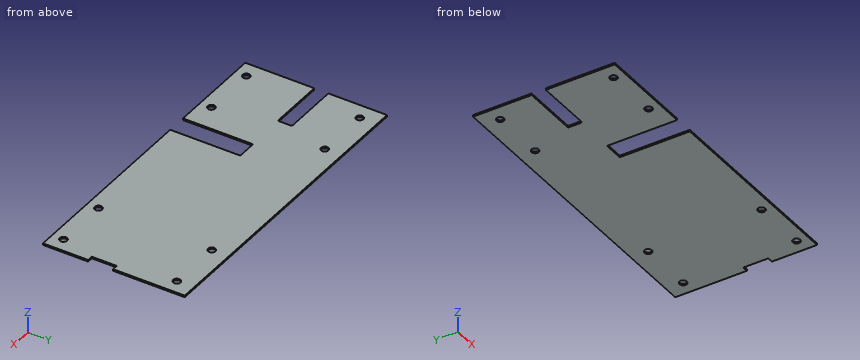
```python
from build123d import *

# Parameters (mm, degrees)
ESQUISSE1_W             = 555
ESQUISSE1_H             = 250
ESQUISSE1_R             = 6.5
BOSS_EXTRU_1_DEPTH      = 3
ESQUISSE4_W             = 100
ESQUISSE4_H             = 25
ESQUISSE4_W_2           = 35
ESQUISSE4_H_2           = 123.628962184
ESQUISSE4_W_3           = 10
ESQUISSE4_H_3           = 44
ENL_V_MAT_EXTRU_3_DEPTH = 10
CONG_1_R                = 2


with BuildPart() as part:
    # Esquisse1 → Boss.-Extru.1 (new body)
    with BuildSketch(Plane.XY):
        Rectangle(ESQUISSE1_W, ESQUISSE1_H)
        with Locations((156.5, 95)):
            Circle(ESQUISSE1_R, mode=Mode.SUBTRACT)
        with Locations((252.5, 95)):
            Circle(ESQUISSE1_R, mode=Mode.SUBTRACT)
        with Locations((156.5, -105)):
            Circle(ESQUISSE1_R, mode=Mode.SUBTRACT)
        with Locations((252.5, -105)):
            Circle(ESQUISSE1_R, mode=Mode.SUBTRACT)
        with Locations((-153.5, -105)):
            Circle(ESQUISSE1_R, mode=Mode.SUBTRACT)
        with Locations((-153.5, 95)):
            Circle(ESQUISSE1_R, mode=Mode.SUBTRACT)
        with Locations((-249.5, 95)):
            Circle(ESQUISSE1_R, mode=Mode.SUBTRACT)
        with Locations((-249.5, -105)):
            Circle(ESQUISSE1_R, mode=Mode.SUBTRACT)
    extrude(amount=BOSS_EXTRU_1_DEPTH)

    # Esquisse4 → Enlèv. mat.-Extru.3 (cut)
    with BuildSketch(Plane.XY.offset(3)):
        with Locations((-227.5, 9.128962184)):
            Rectangle(ESQUISSE4_W, ESQUISSE4_H)
        with Locations((-89, -63.185518908)):
            Rectangle(ESQUISSE4_W_2, ESQUISSE4_H_2)
        with Locations((272.5, -23.371037816)):
            Rectangle(ESQUISSE4_W_3, ESQUISSE4_H_3)
    extrude(amount=-ENL_V_MAT_EXTRU_3_DEPTH, mode=Mode.SUBTRACT)

    # Congé1
    cong_1_edges = [part.edges().sort_by_distance(p)[0] for p in [
        (-177.5, 21.628962184, 1.5),
        (-177.5, -3.371037816, 1.5),
        (-106.5, -1.371037816, 1.5),
        (-71.5, -1.371037816, 1.5),
    ]]
    fillet(cong_1_edges, radius=CONG_1_R)


solid = part.part
```
Geometry: final body of the model. Coordinates: model frame, mm. Give positions to 0.01 mm unless a question says otherwise; leave off trailing zeros. Loops run counter-clockwise (first coordinate to the right, second up) from the corner with the lowest first, then second, coordinate; pieces in that order, holes last. Notation, with made-up numbers: (84.25, 83.5) - (136.25, 83.5) arc R13 cw to (136.25, 93.5) - close; hole circle Ø3 at (20, -32). An arc over 180 degrees is marked (long way). Answer as CSV lines item,"result". Start each with the question number.
(1) Pin query (flat end, axial travel): P1, Ø0.9, axis at y = -23.5, z = 1, coming from the +X side. Return the tip coordinate at first contact, or that it passes through.
(2) Section query A-A (x = 252.5). Output: boundary loops of the cut face in (y, z).
(3) Ray query, line 1 along Y through (x, z) = (-153.5, 1.3); line 2 along Y through (x, z) = (-213.5, 0.9); line 3 along X through (y, z) = (-88, 2.6). Return the intervals inside material, ascending. Write a range as [from, to].
(4) Section query D-D (z = 0.75). Give the number of separate pieces and of enclosed holes in the cut face, and give its area (3 significant figures).
(5) Section query C-C (x = -211.5). Output: boundary loops of the cut face in (y, z), and give its area (3 significant figures).
(6) Section query B-B (y = 95). Output: boundary loops of the cut face in (x, z), and give its area (3 significant figures).
Worked answers:
1,P1,"stops at x = 267.5"
2,outline,"(-125, 0) - (-111.5, 0) - (-111.5, 3) - (-125, 3) - close; (-98.5, 0) - (88.5, 0) - (88.5, 3) - (-98.5, 3) - close; (101.5, 0) - (125, 0) - (125, 3) - (101.5, 3) - close"
3,line 1,"y = [-125, -111.5], [-98.5, 88.5], [101.5, 125]"
3,line 2,"y = [-125, -3.37], [21.63, 125]"
3,line 3,"x = [-277.5, -106.5], [-71.5, 277.5]"
4,separate pieces,"1"
4,enclosed holes,"8"
4,area,"130,000 mm^2"
5,outline,"(-125, 0) - (-3.37, 0) - (-3.37, 3) - (-125, 3) - close; (21.63, 0) - (125, 0) - (125, 3) - (21.63, 3) - close"
5,area,"675 mm^2"
6,outline,"(-277.5, 0) - (-256, 0) - (-256, 3) - (-277.5, 3) - close; (-243, 0) - (-160, 0) - (-160, 3) - (-243, 3) - close; (-147, 0) - (150, 0) - (150, 3) - (-147, 3) - close; (163, 0) - (246, 0) - (246, 3) - (163, 3) - close; (259, 0) - (277.5, 0) - (277.5, 3) - (259, 3) - close"
6,area,"1,510 mm^2"
